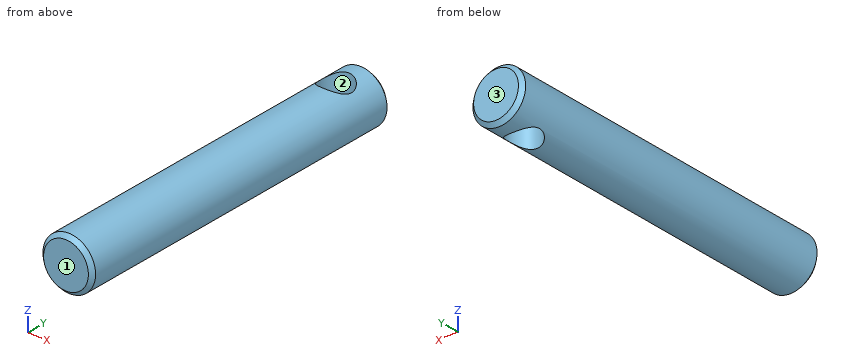
```python
from build123d import *

# Parameters (mm, degrees)
SKETCH1_R               = 13.5
BOSS_EXTRUDE1_DEPTH     = 181
SKETCH2_R               = 8
CUT_EXTRUDE1_DEPTH      = 14.5
CUT_EXTRUDE1_DEPTH_BACK = 14.5
CHAMFER1_SIZE           = 2


with BuildPart() as part:
    # Sketch1 → Boss-Extrude1 (new body)
    with BuildSketch(Plane(origin=(0, 0, 0), x_dir=(1, 0, 0), z_dir=(0, 1, 0))):
        Circle(SKETCH1_R)
    extrude(amount=BOSS_EXTRUDE1_DEPTH)

    # Sketch2 → Cut-Extrude1 (cut, two sides)
    with BuildSketch(Plane.XY) as cut_extrude1_sk:
        with Locations((0, 164)):
            Circle(SKETCH2_R)
    extrude(amount=CUT_EXTRUDE1_DEPTH, mode=Mode.SUBTRACT)
    extrude(cut_extrude1_sk.sketch, amount=-CUT_EXTRUDE1_DEPTH_BACK, mode=Mode.SUBTRACT)

    # Chamfer1
    chamfer1_edges = [part.edges().sort_by_distance(p)[0] for p in [
        (-13.5, 0, 0),
        (-13.5, 181, 0),
    ]]
    chamfer(chamfer1_edges, length=CHAMFER1_SIZE)


solid = part.part
```
Source: CAD feature listing. Evaluate the final solid. Frame: model axes, mm. Face numbers are marked on the shaded views. Coordinates: 2 decimals unless noted, no trailing zeros. Order: outer loops, then holes, each group sorted by start corner. A loop starts at its lowest first (then second) coordinate and runs counter-clockwise, first axis right, second up. Notation, with made-up numbers: M 6,41.5 L 60,41.5 A21 ccw 60,78.5 Z; hole C 4,6 d3. An arc over 180 degrees is marked long. Write each question's results on one line, items separated by ' | '. Start each with the question number.
1) Draft query along Y for the marked faces 1, 2 and 3. Return one class per face: released by +Y, released by -Y, zero draft, split by the parting line, or undercut.
2) Line query: line 1 (Y direction, x = 0, z = 1); line 2 (Y direction, x = 4.5, z = 11); line 3 (X direction, y = 152, z = -0.25). Output: solid intervals per line, ascending. Write a range as from..to.
3) Section query B-B (y = 164). Return the cut outline in (x, z).
4) Section query A-A (z = 0). Return the cut outline in (x, y), plus the area to 3 significant figures.
5) Contact query for flat-ended pins moving along their axis: pin 1 Ø3 at (y, z) = (72, -3) entering from +X; pin 2 Ø5 at (y, z) = (84.5, 3.5) entering from +X. Output: stop coordinate, or through.
Answers:
1) face 1: released by -Y | face 2: undercut | face 3: released by +Y
2) line 1: y = 0..156, 172..181 | line 2: y = 0.38..157.39, 170.61..180.62 | line 3: x = -13.5..13.5
3) outline: M -8,-10.87 L -8,10.87 A13.5 ccw Z; M 8,-10.87 A13.5 ccw 8,10.87 Z
4) outline: M -13.5,2 L -11.5,0 L 11.5,0 L 13.5,2 L 13.5,179 L 11.5,181 L -11.5,181 L -13.5,179 Z; hole C 0,164 d16 | area: 4,680 mm^2
5) pin 1: stops at x = 13.42 | pin 2: stops at x = 13.46
